```python
from build123d import *

# Parameters (mm, degrees)
SKETCH3_R           = 17
BOSS_EXTRUDE1_DEPTH = 40
SKETCH6_R           = 19
BOSS_EXTRUDE2_DEPTH = 8
BOSS_EXTRUDE3_DEPTH = 12
SKETCH8_R           = 16
BOSS_EXTRUDE4_DEPTH = 15


with BuildPart() as part:
    # Sketch3 → Boss-Extrude1 (new body)
    with BuildSketch(Plane.XY):
        Circle(SKETCH3_R)
    extrude(amount=BOSS_EXTRUDE1_DEPTH)

    # Sketch6 → Boss-Extrude2 (add)
    with BuildSketch(Plane.XY.offset(40)):
        Circle(SKETCH6_R)
    extrude(amount=-BOSS_EXTRUDE2_DEPTH)

    # Sketch7 → Boss-Extrude3 (add)
    with BuildSketch(Plane.XY.offset(40)):
        with BuildLine():
            ThreePointArc((-44, -13.416407865), (0, -46), (44, -13.416407865))
            ThreePointArc((44, -13.416407865), (33.683444249, 16.469257624), (13.668094758, 40.943123461))
            ThreePointArc((13.668094758, 40.943123461), (0, 46), (-13.668094758, 40.943123461))
            ThreePointArc((-13.668094758, 40.943123461), (-33.683444249, 16.469257624), (-44, -13.416407865))
        make_face()
    extrude(amount=BOSS_EXTRUDE3_DEPTH)

    # Sketch8 → Boss-Extrude4 (add)
    with BuildSketch(Plane.XY.offset(52)):
        with Locations(Location((0, 25, 0), (0, 0, 180))):
            Circle(SKETCH8_R)
    extrude(amount=BOSS_EXTRUDE4_DEPTH)

    # Mirror2: part across plane


with BuildPart() as part_1:
    add(part.part)
    add(part.part.mirror(Plane(origin=(0, 25, 67), x_dir=(1, 0, 0), z_dir=(0, 0, 1))))


solid = part_1.part
```
The listing builds one solid part. Answer for the finished solid, in the listing's coordinates (mm). A direction names the side the tool comes from. Coordinates: 2 decimals unless noted, no trailing zeros. Loops run counter-clockwise (first coordinate to the right, second up) from the corner with the lowest first, then second, coordinate; pieces in that order, holes last. Notation, with made-up numbers: (49, 23) - (54, 23) arc R19 cw to (54, 32) - close; hole circle Ø2 at (-34, -32). An arc over 180 degrees is marked (long way). Use a Markdown table: item, result. Add a question column.
1) The part is cut by section B-B, the plane x = 24. Give the vertices of the cut face in (y, z), and give its area (3 significant figures).
2) The part is cut by section D-D, the plane y = -38.5. Give the vertices of the cut face in (x, z), and give its area (3 significant figures).
3) The part is cut by section A-A, the plane y = -5. Give the vertices of the cut face in (x, z).
4) Find the intervals of material crossed by line 1 (Z direction, x = -32.5, y = -15); line 2 (Y direction, x = 1, z = 92.5); line 3 (Z direction, x = -2.5, y = -17), in increasing order.
5) The mould has two halves that part along Z. Classify faces 1 (the flat face through (-14, -10, 102)), 2 (the cylindrical face through (0, 46, 88)), 3 (the flat face through (-1, -10, 52)), 4 (the flat face through (-1, -10, 82)): released by +Z, released by -Z, zero draft, split by the parting line, or undercut.
6) For faces 5 (the cylindrical face through (9.139, 14.334, 118.224)), 6 (the cylindrical face through (-33.466, 16.857, 88.084)), 7 (the flat face through (-1, -20, 40)), determine the directions among +Z, -Z, +X, -X, +Y, -Y from which every point of the face is accessible in a straight line to the end or side of a thin tool.
7) The part is cut by section C-C, the plane x = 0. Give the vertices of the cut face in (y, z), and give its area (3 significant figures).
8) Given pin 1 (10 mm diameter, centred on x = 27.5, z = 61.5, fed in from -Y); pin 2 (1 mm diameter, centred on x = -6, y = 17.5, fed in from -Z); pin 3 (10 mm diameter, centred on x = 15, z = 26, fed in from +Y); pin 4 (1.5 mm diameter, centred on x = -29, y = -32.5, fed in from +Z), each flat-ended and moving along its own axis, determine where each tip first touches the part or whether it passes through.
Here are the results:
| question | item | result |
|---|---|---|
| 1 | outline | (-39.24, 40) - (30.51, 40) - (30.51, 52) - (-39.24, 52) - close; (-39.24, 82) - (30.51, 82) - (30.51, 94) - (-39.24, 94) - close |
| 1 | area | 1,670 mm^2 |
| 2 | outline | (-25.17, 40) - (25.17, 40) - (25.17, 52) - (-25.17, 52) - close; (-25.17, 82) - (25.17, 82) - (25.17, 94) - (-25.17, 94) - close |
| 2 | area | 1,210 mm^2 |
| 3 | outline | (-42.26, 40) - (-18.33, 40) - (-18.33, 32) - (-16.25, 32) - (-16.25, 0) - (16.25, 0) - (16.25, 32) - (18.33, 32) - (18.33, 40) - (42.26, 40) - (42.26, 52) - (-42.26, 52) - close; (-42.26, 82) - (42.26, 82) - (42.26, 94) - (18.33, 94) - (18.33, 102) - (16.25, 102) - (16.25, 134) - (-16.25, 134) - (-16.25, 102) - (-18.33, 102) - (-18.33, 94) - (-42.26, 94) - close |
| 4 | line 1 | z = 40 to 52, 82 to 94 |
| 4 | line 2 | y = -45.99 to 45.98 |
| 4 | line 3 | z = 32 to 52, 82 to 102 |
| 5 | face 1 | released by +Z |
| 5 | face 2 | zero draft |
| 5 | face 3 | undercut |
| 5 | face 4 | undercut |
| 6 | face 5 | +Z |
| 6 | face 6 | +Z, -Z, -X, +Y |
| 6 | face 7 | -Z |
| 7 | outline | (-46, 40) - (-19, 40) - (-19, 32) - (-17, 32) - (-17, 0) - (17, 0) - (17, 32) - (19, 32) - (19, 40) - (46, 40) - (46, 52) - (41, 52) - (41, 82) - (46, 82) - (46, 94) - (19, 94) - (19, 102) - (17, 102) - (17, 134) - (-17, 134) - (-17, 102) - (-19, 102) - (-19, 94) - (-46, 94) - (-46, 82) - (9, 82) - (9, 52) - (-46, 52) - close |
| 7 | area | 5,950 mm^2 |
| 8 | pin 1 | passes through |
| 8 | pin 2 | stops at z = 32 |
| 8 | pin 3 | stops at y = 13.75 |
| 8 | pin 4 | stops at z = 94 |
